Input: part model. Units: mm. Frame: model coordinates. Round coordinates to 2 decimals unless told otherwise and drop trailing zeros. Order: outer loops, then holes, each group sorted by start corner. A loop starts at its lowest first (then second) coordinate and runs counter-clockwise, first axis right, second up. Notation, with made-up numbers: (-3, 35) - (41, 35) arc R7 cw to (41, 42) - close; hole circle Ø1 at (21, 81.5). An arc over 180 degrees is marked (long way). One line per item, written item: value. Start each with the question number.
from build123d import *

# Parameters (mm, degrees)
SKETCH_1_W     = 0.64
SKETCH_1_H     = 0.64
CHAMFER_1_SIZE = 0.1


with BuildPart() as part:
    # По траектории1: sweep along a path in Эскиз2
    with BuildLine(Plane.XY) as sweep_1_path:
        Line((0, 0), (0, 6.28))
        ThreePointArc((0, 6.28), (0.146446609, 6.633553391), (0.5, 6.78))
        Line((0.5, 6.78), (6.78, 6.78))
    # Эскиз1 → По траектории1 (sweep)
    with BuildSketch(Plane(origin=(0, 0, 0), x_dir=(1, 0, 0), z_dir=(0, 1, 0))):
        Rectangle(SKETCH_1_W, SKETCH_1_H)
    sweep(path=sweep_1_path.line)

    # Фаска1
    chamfer_1_edges = [part.edges().sort_by_distance(p)[0] for p in [
        (6.78, 6.78, 0.32),
        (6.78, 7.1, 0),
        (6.78, 6.78, -0.32),
        (0, 0, 0.32),
        (-0.32, 0, 0),
        (0, 0, -0.32),
        (0.32, 0, 0),
    ]]
    chamfer(chamfer_1_edges, length=CHAMFER_1_SIZE)


solid = part.part
Item 1: Section query A-A on z = 0.05. Return loops of the section in (x, y), and give its area (3 significant figures).
Item 2: Line query: L1, parallel to X at y = 2, z = 0.2; L2, parallel to Y at x = 3.5, z = -0.05; L3, parallel to X at y = 6.5, z = -0.2. Output: solid intervals per line, ascending.
Item 3: Section query C-C on x = 5.25. Return loops of the section in (y, z), and give its area (3 significant figures).
Item 4: Section query B-B on y = 0.5. Return loops of the section in (x, z).
Geometry results:
1. outline: (-0.32, 0.1) - (-0.22, 0) - (0.22, 0) - (0.32, 0.1) - (0.32, 6.28) arc R0.18 cw to (0.5, 6.46) - (6.78, 6.46) - (6.78, 7) - (6.68, 7.1) - (0.5, 7.1) arc R0.82 ccw to (-0.32, 6.28) - close
1. area: 8.53 mm^2
2. L1: x = -0.32 to 0.32
2. L2: y = 6.46 to 7.1
2. L3: x = -0.29 to 6.78
3. outline: (6.46, -0.32) - (7.1, -0.32) - (7.1, 0.32) - (6.46, 0.32) - close
3. area: 0.410 mm^2
4. outline: (-0.32, -0.32) - (0.32, -0.32) - (0.32, 0.32) - (-0.32, 0.32) - close
